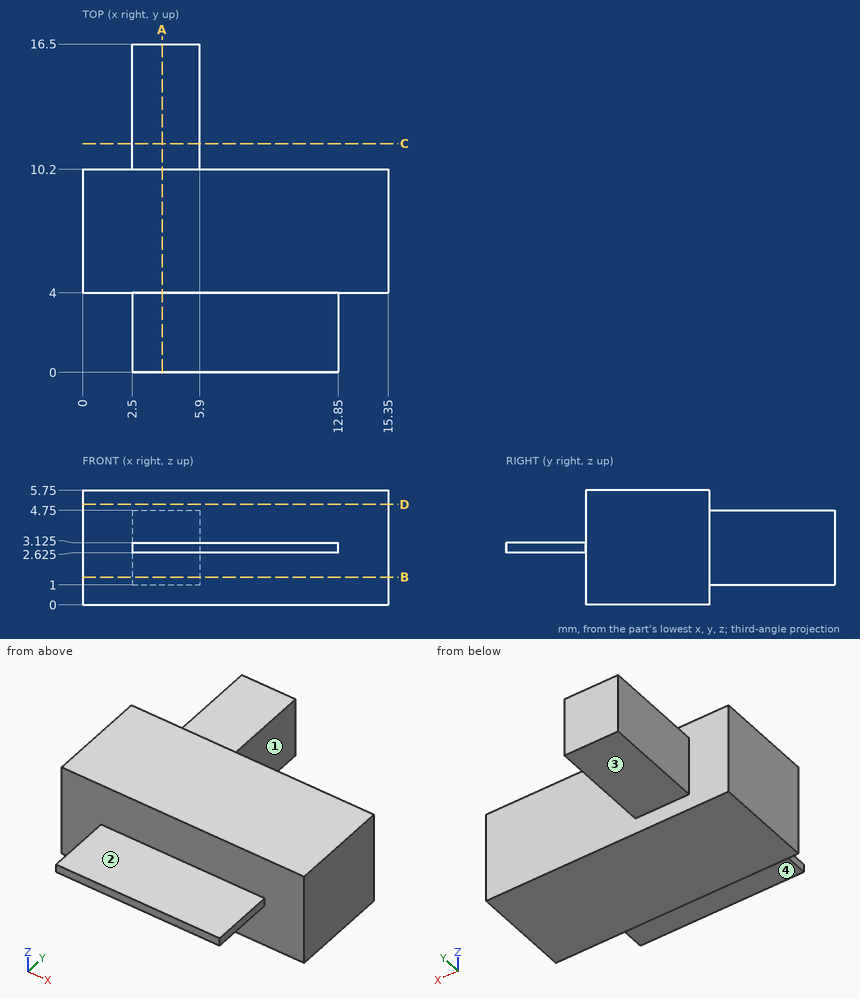
Could you check a few things on this drawing? It's one solid part, dimensions in mm from its lowest x, y, z. A direction names the side the tool comes from. Round coordinates to 2 decimals unless told otherwise and drop trailing zeros. Write each loop counter-clockwise with the first axis right and the second up, starting at its lowest first coordinate (ties: lowest second). Pieces come first, ordered by that corner, then holes.
Q1. If we section it at B-B on z = 1.4: Write out the boundary of the cut face in (x, y), plus the area to 3 significant figures.
Q2. Please list where these lines run through material, in increasing order: probe 1 along Y at (x, z) = (4, 1.1); probe 2 along Y at (x, z) = (10.75, 0.35); probe 3 along Z at (x, y) = (7, 2.5) (3 decimals).
Q3. Which directions (+Z, -Z, +X, -X, +Y, -Y) give clear straight access to the entire face, cutting with the end or side of a thin tool? Please do the marked faces 1, 2, 3 and 4.
Q4. Will these pins go through, and if not, where does the flat tip stop? P1, Ø3, axis at x = 11, y = 13.5, coming from the -Z side; P2, Ø3, axis at x = 8.5, z = 3.5, coming from the +Y side; P3, Ø1, axis at x = 4, y = 12, coming from the -Z side; P4, Ø1.2, axis at x = 8, y = 2.5, coming from the -Z side (3 decimals).
Q5. If we section it at C-C on y = 11.5: Write out the boundary of the cut face in (x, z), plus the area to 4 significant figures.
Q6. If we section it at D-D on z = 5.05: Write out the boundary of the cut face in (x, y).
Q7. If we section it at A-A on x = 4: Write out the boundary of the cut face in (y, z) (3 decimals).
Answer below:
1. outline: (0, 4) - (15.35, 4) - (15.35, 10.2) - (5.9, 10.2) - (5.9, 16.5) - (2.5, 16.5) - (2.5, 10.2) - (0, 10.2) - close
1. area: 117 mm2
2. probe 1: y = 4 to 16.5
2. probe 2: y = 4 to 10.2
2. probe 3: z = 2.625 to 3.125
3. face 1: +Z, -Z, +X, +Y
3. face 2: +Z, +X, -X, -Y
3. face 3: -Z, +X, -X, +Y
3. face 4: -Z, +X, -X, -Y
4. P1: passes through
4. P2: stops at y = 10.2
4. P3: stops at z = 1
4. P4: stops at z = 2.625
5. outline: (2.5, 1) - (5.9, 1) - (5.9, 4.75) - (2.5, 4.75) - close
5. area: 12.75 mm2
6. outline: (0, 4) - (15.35, 4) - (15.35, 10.2) - (0, 10.2) - close
7. outline: (0, 2.625) - (4, 2.625) - (4, 0) - (10.2, 0) - (10.2, 1) - (16.5, 1) - (16.5, 4.75) - (10.2, 4.75) - (10.2, 5.75) - (4, 5.75) - (4, 3.125) - (0, 3.125) - close
